Can you work these out from the drawing? Everything is in mm from the part's minimum corner. A direction names the side the tool comes from. Round coordinates to 2 decimals unless told otherwise and drop trailing zeros. Loops run counter-clockwise (first coordinate to the right, second up) from the corner with the lowest first, then second, coordinate; pieces in that order, holes last. Notation, with made-up numbers: (21.25, 9.5) -> (80.25, 9.5) arc R16 ccw to (80.25, 22.5) -> close; hole circle Ø2 at (81.25, 26). An arc over 180 degrees is marked (long way). One line per item, written item: value.
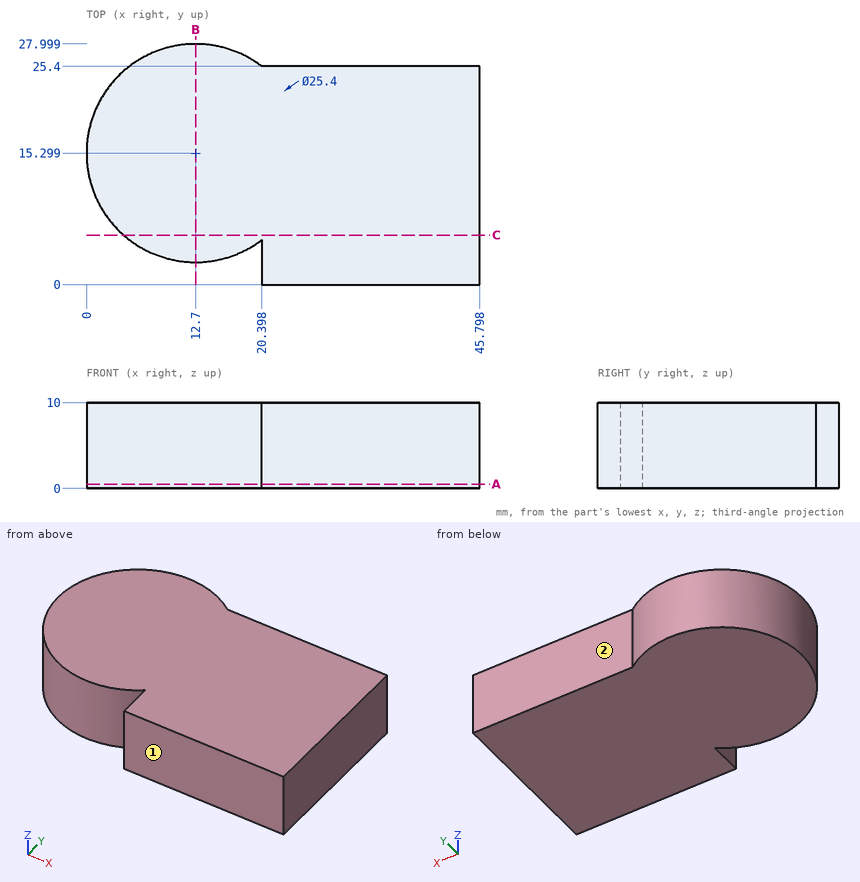
(1) If I drill on L1, parallel to Y at x = 30.5, z = 7.25; L2, parallel to Y at x = 13, z = 8.25; L3, parallel to X at y = 10.75, z = 7.75, over which ranges is the centre line in solid material (lowest first)?
Recorded:
L1: 0 to 25.4
L2: 2.6 to 28
L3: 0.84 to 45.8
(2) If we section it at C-C, the plane y = 5.75: Please give me the cut outline in (x, z), then the cut area to 3 significant figures.
Recorded:
outline: (4.33, 0) -> (45.8, 0) -> (45.8, 10) -> (4.33, 10) -> close
area: 415 mm²
(3) If we section it at A-A, the plane z = 0.5: Please give me the cut outline in (x, y).
Recorded:
outline: (20.4, 0) -> (45.8, 0) -> (45.8, 25.4) -> (20.4, 25.4) arc R12.7 ccw (long way) to (20.4, 5.2) -> close
(4) I'm going to push flat-ended pins straight in: pin 1 Ø6 at (x, y) = (39.5, 19.5) entering from -Z; pin 2 Ø3 at (x, z) = (39, 4) entering from +Y; pin 3 Ø2.5 at (y, z) = (3, 6.5) entering from -X. Where does each tip first touch, or does it pass through?
Recorded:
pin 1: z = 0
pin 2: y = 25.4
pin 3: x = 6.44
(5) For the marked faces 1 and 2, which set-ups out of +Z, -Z, +X, -X, +Y, -Y let a thin tool reach every point of the face, with its end or its side?
Recorded:
face 1: +Z, -Z, +X, -X, -Y
face 2: +Z, -Z, +X, +Y
(6) If we section it at B-B, the plane x = 12.7: Please give me the cut outline in (y, z), then the cut area to 3 significant figures.
Recorded:
outline: (2.6, 0) -> (28, 0) -> (28, 10) -> (2.6, 10) -> close
area: 254 mm²
